from build123d import *

# Parameters (mm, degrees)
SKETCH1_W           = 8.24
SKETCH1_H           = 15
BOSS_EXTRUDE1_DEPTH = 3.7
BOSS_EXTRUDE2_DEPTH = 5
SKETCH3_W           = 0.5
SKETCH3_H           = 0.25
BOSS_EXTRUDE3_DEPTH = 3.1


with BuildPart() as part:
    # Sketch1 → Boss-Extrude1 (new body)
    with BuildSketch(Plane(origin=(0, 0, 0), x_dir=(1, 0, 0), z_dir=(0, 1, 0))):
        with Locations((-16.236881088, -0.721940399)):
            Rectangle(SKETCH1_W, SKETCH1_H)
    extrude(amount=BOSS_EXTRUDE1_DEPTH)

    # Sketch2 → Boss-Extrude2 (add)
    with BuildSketch(Plane(origin=(0, 3.7, 0), x_dir=(1, 0, 0), z_dir=(0, 1, 0))):
        Polygon((-20.356881088, -8.221940399), (-12.116881088, -8.221940399), (-10.756881088, -8.221940399), (-10.756881088, 6.778059601), (-12.116881088, 6.778059601), (-20.356881088, 6.778059601), align=None)
    extrude(amount=BOSS_EXTRUDE2_DEPTH)

    # Sketch3 → Boss-Extrude3 (add)
    with BuildSketch(Plane(origin=(-10.756881088, 0, 0), x_dir=(0, 0, -1), z_dir=(1, 0, 0))):
        with Locations((-5.721940399, 6.2)):
            Rectangle(SKETCH3_W, SKETCH3_H)
        with Locations((-3.221940399, 6.2)):
            Rectangle(SKETCH3_W, SKETCH3_H)
        with Locations((-0.721940399, 6.2)):
            Rectangle(SKETCH3_W, SKETCH3_H)
        with Locations((1.778059601, 6.2)):
            Rectangle(SKETCH3_W, SKETCH3_H)
        with Locations((4.278059601, 6.2)):
            Rectangle(SKETCH3_W, SKETCH3_H)
    extrude(amount=BOSS_EXTRUDE3_DEPTH)


solid = part.part
Geometry check sheet. Reference: the model listing, model coordinates, mm. A direction names the side the tool comes from. Coordinates: 2 decimals unless noted, no trailing zeros. Order: outer loops, then holes, each group sorted by start corner. A loop starts at its lowest first (then second) coordinate and runs counter-clockwise, first axis right, second up. Notation, with made-up numbers: (71, 19) -> (102, 19) arc R20 cw to (102, 52) -> close; hole circle Ø2 at (28, 50). An arc over 180 degrees is marked (long way). Use a Markdown table: item, result. Add a question column.
1. Cross-section at A-A (x = -8.25). Enter the section's corners in (y, z) (3 decimals).
2. Set-up check for faces 1 (the face through (-11, 3.7, 1)), 2 (the face through (-16, 0, 1)): record each of +Z, -Z, +X, -X, +Y, -Y from which the full face is reachable in a straight line by a thin tool's end or side.
3. Go/stop test with flat-tipped pins: pin 1 Ø1.1 at (x, z) = (-11, 0.5) entering from -Y; pin 2 Ø0.6 at (x, z) = (-8.5, -4) entering from -Y (3 decimals); pin 3 Ø4 at (x, z) = (-13.5, -3) entering from -Y; pin 4 Ø1.5 at (x, y) = (-9.5, 6) entering from -Z. Record where each tip stops, or that it passes through.
4. Cross-section at B-B (z = 3.25). Enter the section's corners in (x, y) (3 decimals), and give its area (3 significant figures).
5. Cross-section at C-C (y = 3.25). Enter the section's corners in (x, z).
6. Cross-section at D-D (z = -5.75). Enter the section's corners in (x, y), and give its area (3 significant figures).
7. Material ranges on L1, parallel to X at y = 1.5, z = 6; L2, parallel to X at y = 8.25, z = 5.25, recorded low to high.
Filled sheet:
| question | item | result |
|---|---|---|
| 1 | outline | (6.075, -4.528) -> (6.325, -4.528) -> (6.325, -4.028) -> (6.075, -4.028) -> close; (6.075, -2.028) -> (6.325, -2.028) -> (6.325, -1.528) -> (6.075, -1.528) -> close; (6.075, 0.472) -> (6.325, 0.472) -> (6.325, 0.972) -> (6.075, 0.972) -> close; (6.075, 2.972) -> (6.325, 2.972) -> (6.325, 3.472) -> (6.075, 3.472) -> close; (6.075, 5.472) -> (6.325, 5.472) -> (6.325, 5.972) -> (6.075, 5.972) -> close |
| 2 | face 1 | +Z, -Z, +X, -Y |
| 2 | face 2 | +Z, -Z, +X, -X, -Y |
| 3 | pin 1 | y = 3.7 |
| 3 | pin 2 | y = 6.075 |
| 3 | pin 3 | y = 0 |
| 3 | pin 4 | z = -4.53 |
| 4 | outline | (-20.357, 0) -> (-12.117, 0) -> (-12.117, 3.7) -> (-10.757, 3.7) -> (-10.757, 6.075) -> (-7.657, 6.075) -> (-7.657, 6.325) -> (-10.757, 6.325) -> (-10.757, 8.7) -> (-20.357, 8.7) -> close |
| 4 | area | 79.3 mm2 |
| 5 | outline | (-20.36, -6.78) -> (-12.12, -6.78) -> (-12.12, 8.22) -> (-20.36, 8.22) -> close |
| 6 | outline | (-20.36, 0) -> (-12.12, 0) -> (-12.12, 3.7) -> (-10.76, 3.7) -> (-10.76, 8.7) -> (-20.36, 8.7) -> close |
| 6 | area | 78.5 mm2 |
| 7 | L1 | -20.36 to -12.12 |
| 7 | L2 | -20.36 to -10.76 |
